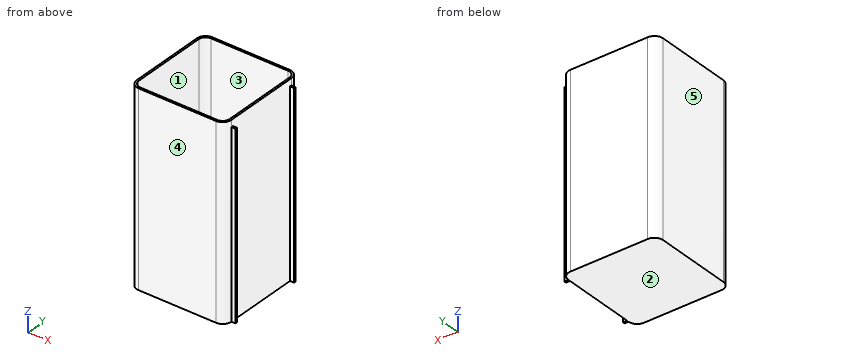
from build123d import *

# Parameters (mm, degrees)
SKETCH1_W           = 70
SKETCH1_H           = 70
BOSS_EXTRUDE1_DEPTH = 140
SKETCH2_W           = 67.2
SKETCH2_H           = 67.2
CUT_EXTRUDE1_DEPTH  = 138.4
FILLET1_R           = 5
FILLET2_R           = 6.4
SKETCH3_W           = 135
SKETCH3_H           = 1.5
BOSS_EXTRUDE2_DEPTH = 3


with BuildPart() as part:
    # Sketch1 → Boss-Extrude1 (new body)
    with BuildSketch(Plane.XY):
        with Locations((35, 35)):
            Rectangle(SKETCH1_W, SKETCH1_H)
    extrude(amount=BOSS_EXTRUDE1_DEPTH)

    # Sketch2 → Cut-Extrude1 (cut)
    with BuildSketch(Plane.XY.offset(140)):
        with Locations((35, 35)):
            Rectangle(SKETCH2_W, SKETCH2_H)
    extrude(amount=-CUT_EXTRUDE1_DEPTH, mode=Mode.SUBTRACT)

    # Fillet1
    fillet1_edges = [part.edges().sort_by_distance(p)[0] for p in [
        (1.4, 1.4, 70.8),
        (1.4, 68.6, 70.8),
        (68.6, 68.6, 70.8),
        (68.6, 1.4, 70.8),
    ]]
    fillet(fillet1_edges, radius=FILLET1_R)

    # Fillet2
    fillet2_edges = [part.edges().sort_by_distance(p)[0] for p in [
        (0, 70, 70),
        (70, 70, 70),
        (70, 0, 70),
        (0, 0, 70),
    ]]
    fillet(fillet2_edges, radius=FILLET2_R)

    # Sketch3 → Boss-Extrude2 (add)
    with BuildSketch(Plane(origin=(70, 0, 0), x_dir=(0, 0, -1), z_dir=(1, 0, 0))):
        with Locations((-67.5, 7.15)):
            Rectangle(SKETCH3_W, SKETCH3_H)
        with Locations((-67.5, 62.85)):
            Rectangle(SKETCH3_W, SKETCH3_H)
    extrude(amount=BOSS_EXTRUDE2_DEPTH)


solid = part.part
The listing builds one solid part. Answer for the finished solid, in the listing's coordinates (mm). Face numbers are marked on the shaded views. A direction names the side the tool comes from. Coordinates: 2 decimals unless noted, no trailing zeros. Order: outer loops, then holes, each group sorted by start corner. A loop starts at its lowest first (then second) coordinate and runs counter-clockwise, first axis right, second up. Notation, with made-up numbers: (67.25, 17.25) -> (73.25, 17.25) arc R26 cw to (73.25, 54.25) -> close; hole circle Ø5 at (24.5, 70.25). An arc over 180 degrees is marked (long way). Answer in a Markdown table with one row per item. Add a question column.
Item 1: Which of the six approach directions +Z, -Z, +X, -X, +Y, -Y give full straight-line access (tool end or side, diameter ignored) to the marked faces 1 and 2?
Item 2: Find section A-A (z = 126.5). Write down the section's boundary in (x, y).
Item 3: Each of these flat-tipped pins is pushed along its axis until it touches: P1, Ø5, axis at y = 21.5, z = 66.5, coming from the +X side; P2, Ø1.5, axis at x = 71.5, z = 81, coming from the -Y side; P3, Ø0.8, axis at x = 71.5, y = 7.5, coming from the +Z side. Where does it stop, or does it pass through?
Item 4: Determine the mould class of the marked faces 3, 4 and 5 for opening direction X: +X half, -X half, draft (parallel to the pull), parting line (faces both ways), or undercut.
Item 5: Find the intervals of material crossed by L1, parallel to Y at x = 28, z = 121.5; L2, parallel to Y at x = 70.5, z = 85.5, in increasing order. Write a range as from..to.
Item 6: Find section B-B (y = 37). Write down the section's boundary in (x, z), then the cut area to 3 significant figures.
Result set:
| question | item | result |
|---|---|---|
| 1 | face 1 | +Z |
| 1 | face 2 | -Z, +X, -X, +Y, -Y |
| 2 | outline | (0, 6.4) arc R6.4 ccw to (6.4, 0) -> (63.6, 0) arc R6.4 ccw to (70, 6.4) -> (73, 6.4) -> (73, 7.9) -> (70, 7.9) -> (70, 62.1) -> (73, 62.1) -> (73, 63.6) -> (70, 63.6) arc R6.4 ccw to (63.6, 70) -> (6.4, 70) arc R6.4 ccw to (0, 63.6) -> close; hole (1.4, 6.4) arc R5 ccw to (6.4, 1.4) -> (63.6, 1.4) arc R5 ccw to (68.6, 6.4) -> (68.6, 63.6) arc R5 ccw to (63.6, 68.6) -> (6.4, 68.6) arc R5 ccw to (1.4, 63.6) -> close |
| 3 | P1 | stops at x = 70 |
| 3 | P2 | stops at y = 6.4 |
| 3 | P3 | stops at z = 135 |
| 4 | face 3 | undercut |
| 4 | face 4 | draft |
| 4 | face 5 | -X half |
| 5 | L1 | y = 0..1.4, 68.6..70 |
| 5 | L2 | y = 6.4..7.9, 62.1..63.6 |
| 6 | outline | (0, 0) -> (70, 0) -> (70, 140) -> (68.6, 140) -> (68.6, 1.6) -> (1.4, 1.6) -> (1.4, 140) -> (0, 140) -> close |
| 6 | area | 500 mm² |
